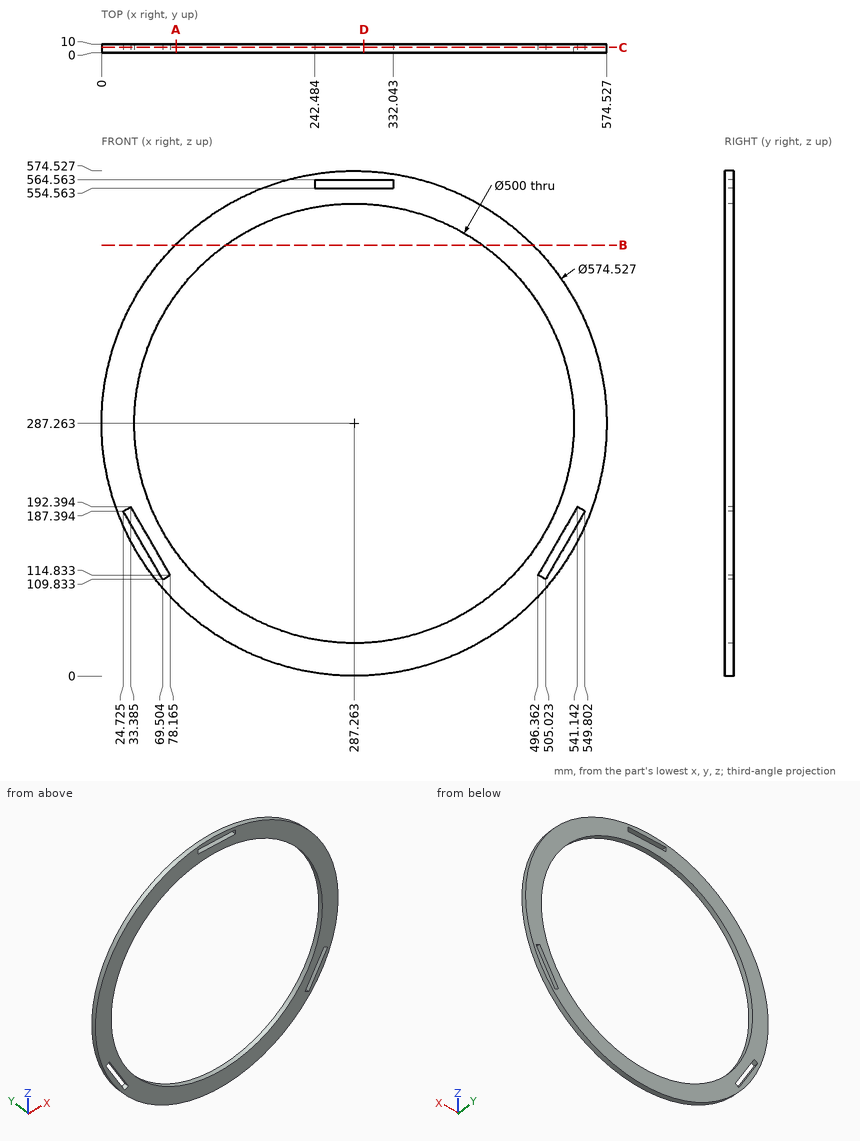
Input: dimensioned drawing with shaded views. Units: mm. Origin: part minimum x, y, z. Round coordinates to 2 decimals unless told otherwise and drop trailing zeros. Loops run counter-clockwise (first coordinate to the right, second up) from the corner with the lowest first, then second, coordinate; pieces in that order, holes last. Notation, with made-up numbers: M 14.25,1.5 L 26.25,1.5 A10 cw 26.25,15.5 Z; hole C -18.75,82 d4. An arc over 180 degrees is marked long. Return JSON: item names as keys, results as strings. Group by question number.
1. Material intervals for line 1 along X through (y, z) = (6, 159) (1 decimal); line 2 along Z through (x, y) = (73.5, 2) (1 decimal); line 3 along X through (y, z) = (3.25, 292), sorted ascending. Write a range as from..to.
2. Section query D-D on x = 298.5. Output: boundary loops of the cut face in (y, z), and give its area (3 significant figures).
3. Section query C-C on y = 6.25. Output: boundary loops of the cut face in (x, z) (1 decimal), and give its area (3 significant figures).
4. Section query A-A on x = 85. Output: boundary loops of the cut face in (y, z), and give its area (3 significant figures).
5. Section query B-B on z = 490. Output: boundary loops of the cut face in (x, y), and give its area (3 significant figures).
6. Pin query (flat end, axial travel): pin 1 (2 mm diameter, centred on y = 7, z = 412, fed in from -X) (1 decimal); pin 2 (4 mm diameter, centred on y = 2.5, z = 129.5, fed in from -X). Return the tip coordinate at first contact, or that it passes through.
Checks:
{
 "1": {"line 1": "x = 30.2..41.1, 52.7..72.7, 501.9..521.9, 533.4..544.3", "line 2": "z = 95.4..112.1, 122.9..157.6, 416.9..479.2", "line 3": "x = 0.04..37.31, 537.22..574.49"},
 "2": {"outline": "M 0,0.22 L 10,0.22 L 10,37.52 L 0,37.52 Z; M 0,537.01 L 10,537.01 L 10,554.56 L 0,554.56 Z; M 0,564.56 L 10,564.56 L 10,574.31 L 0,574.31 Z", "area": "646 mm²"},
 "3": {"outline": "C 287.3,287.3 d574.5; hole M 24.7,187.4 L 69.5,109.8 L 78.2,114.8 L 33.4,192.4 Z; hole C 287.3,287.3 d500; hole M 242.5,554.6 L 332,554.6 L 332,564.6 L 242.5,564.6 Z; hole M 496.4,114.8 L 505,109.8 L 549.8,187.4 L 541.1,192.4 Z", "area": "60,200 mm²"},
 "4": {"outline": "M 0,83.28 L 10,83.28 L 10,140.33 L 0,140.33 Z; M 0,434.2 L 10,434.2 L 10,491.25 L 0,491.25 Z", "area": "1,140 mm²"},
 "5": {"outline": "M 83.75,0 L 140.98,0 L 140.98,10 L 83.75,10 Z; M 433.54,0 L 490.78,0 L 490.78,10 L 433.54,10 Z", "area": "1,140 mm²"},
 "6": {"pin 1": "stops at x = 28", "pin 2": "stops at x = 45.9"}
}
